Check sheet for the modelled part. Datum: model origin and axes. Units: mm. A direction names the side the tool comes from. Give positions to 0.01 mm unless a question says otherwise; leave off trailing zeros. Write each loop counter-clockwise with the first axis right and the second up, starting at its lowest first coordinate (ties: lowest second). Pieces come first, ordered by that corner, then holes. Notation, with made-up numbers: (62, -0.5) -> (84, -0.5) arc R20 cw to (84, 7.5) -> close; hole circle Ø8 at (20, 20). An arc over 180 degrees is marked (long way). Write each question's results on one line, items separated by ' | '. Start each with the question number.
```python
from build123d import *

# Parameters (mm, degrees)
PAD_DEPTH     = 10
SKETCH001_R   = 8
PAD001_DEPTH  = 24
SKETCH002_R   = 5
SKETCH002_R_2 = 2
POCKET_DEPTH  = 34.001


with BuildPart() as part:
    # Sketch → Pad (new body)
    with BuildSketch(Plane.XY):
        with BuildLine():
            ThreePointArc((-13.228757, 9), (-16, 0), (-13.228757, -9))
            Line((-13.228757, -9), (13.228757, -9))
            ThreePointArc((13.228757, -9), (16, 0), (13.228757, 9))
            Line((-13.228757, 9), (13.228757, 9))
        make_face()
    extrude(amount=PAD_DEPTH)

    # Sketch001 (on Face5 of Pad) → Pad001 (join)
    with BuildSketch(Plane(origin=(0, 0, 0), x_dir=(1, 0, 0), z_dir=(0, 0, -1))):
        Circle(SKETCH001_R)
    extrude(amount=PAD001_DEPTH)

    # Sketch002 (on Face5 of Pad001) → Pocket (cut, through all)
    with BuildSketch(Plane.XY.offset(10)):
        Circle(SKETCH002_R)
        with Locations((12, 0)):
            Circle(SKETCH002_R_2)
        with Locations((-12, 0)):
            Circle(SKETCH002_R_2)
    extrude(amount=-POCKET_DEPTH, mode=Mode.SUBTRACT)


solid = part.part
```
Item 1: Mould release check, pull along Y, two halves, no side actions. Record for faces 1 (the flat face through (3.3, 4.1, 10)), 2 (the cylindrical face through (-1.08, -4.88, -6.76)), 3 (the flat face through (0, 9, 5)), 4 (the cylindrical face through (10.4, -1.2, 5.1)): pulls with the +Y half, pulls with the -Y half, needs draft (parallel to the pull), parting line crosses it, or undercut.
Item 2: Thickness scan on probe 1 along Y at (x, z) = (-12, 3.25); probe 2 along Y at (x, z) = (0, 3); probe 3 along Z at (x, y) = (-5, -6.75). Record the ranges inside material, lowest first. Write a range as from..to.
Item 3: Section check C-C on z = -19. Record the boundary of the cut face in (x, y).
Item 4: Depth check by flat-ended pin: pin 1 Ø1 at (y, z) = (-4.5, -14) entering from +X; pin 2 Ø6 at (x, z) = (-9.5, -3.5) entering from +Y; pin 3 Ø5 at (x, y) = (-12, 0) entering from -Z. Enter the tip coordinate at first touch or a pass-through.
Item 5: Set-up check for faces 5 (the cylindrical face through (-1.73, 7.81, -11.83)), 6 (the flat face through (5.2, -0.1, -24)): record each of +Z, -Z, +X, -X, +Y, -Y from which the full face is reachable in a straight line by a thin tool's end or side.
Item 6: Section check D-D on y = 4. Record the boundary of the cut face in (x, z).
Item 7: Section check B-B on y = 0. Record the boundary of the cut face in (x, z), then the cut area to 3 significant figures.
Item 8: Section check A-A on x = -12. Record the boundary of the cut face in (y, z), then the cut area to 3 significant figures.
Check sheet entries:
1) face 1: needs draft | face 2: undercut | face 3: pulls with the +Y half | face 4: undercut
2) probe 1: y = -9..-2, 2..9 | probe 2: y = -9..-5, 5..9 | probe 3: z = 0..10
3) outline: circle Ø16 at (0, 0); hole circle Ø10 at (0, 0)
4) pin 1: stops at x = 6.93 | pin 2: stops at y = 4.66 | pin 3: stops at z = 0
5) face 5: -Z | face 6: -Z, +X, -X, +Y, -Y
6) outline: (-15.49, 0) -> (-6.93, 0) -> (-6.93, -24) -> (-3, -24) -> (-3, 10) -> (-15.49, 10) -> close; (3, -24) -> (6.93, -24) -> (6.93, 0) -> (15.49, 0) -> (15.49, 10) -> (3, 10) -> close
7) outline: (-16, 0) -> (-14, 0) -> (-14, 10) -> (-16, 10) -> close; (-10, 0) -> (-8, 0) -> (-8, -24) -> (-5, -24) -> (-5, 10) -> (-10, 10) -> close; (5, -24) -> (8, -24) -> (8, 0) -> (10, 0) -> (10, 10) -> (5, 10) -> close; (14, 0) -> (16, 0) -> (16, 10) -> (14, 10) -> close | area: 284 mm^2
8) outline: (-9, 0) -> (-2, 0) -> (-2, 10) -> (-9, 10) -> close; (2, 0) -> (9, 0) -> (9, 10) -> (2, 10) -> close | area: 140 mm^2
